Part model, mm, in its own coordinate system. Face numbers are marked on the shaded views. A direction names the side the tool comes from. Give positions to 0.01 mm unless a question says otherwise; leave off trailing zeros. Write each loop counter-clockwise with the first axis right and the second up, starting at its lowest first coordinate (ties: lowest second). Pieces come first, ordered by that corner, then holes. Notation, with made-up numbers: (57, 73.25) - (78, 73.25) arc R27 cw to (78, 91.25) - close; hole circle Ø3 at (55.5, 9.25). An arc over 180 degrees is marked (long way). Answer as a JSON object with one key per item and string values. Group by question number.
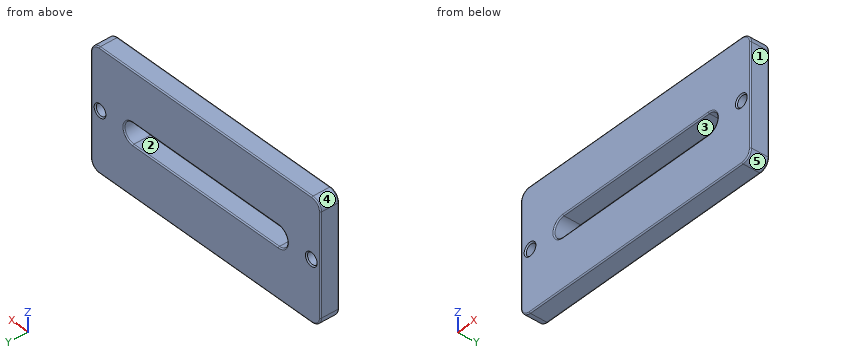
```python
from build123d import *

# Parameters (mm, degrees)
SKETCH1_W           = 82
SKETCH1_H           = 37.8
SKETCH1_R           = 1.75
BOSS_EXTRUDE1_DEPTH = 5.85
FILLET2_R           = 3
FILLET3_R           = 0.35
CHAMFER1_SIZE       = 0.35


with BuildPart() as part:
    # Sketch1 → Boss-Extrude1 (new body)
    with BuildSketch(Plane(origin=(0, 0, 0), x_dir=(1, 0, 0), z_dir=(0, 1, 0))):
        Rectangle(SKETCH1_W, SKETCH1_H)
        with Locations(Location((37.75, 0, 0), (0, 0, 270))):
            Circle(SKETCH1_R, mode=Mode.SUBTRACT)
        with Locations(Location((-37.75, 0, 0), (0, 0, 270))):
            Circle(SKETCH1_R, mode=Mode.SUBTRACT)
        with BuildLine():
            Line((-25.9975, 3.225), (-13.623486154, 3.225))
            Line((-13.623486154, 3.225), (13.623486154, 3.225))
            Line((13.623486154, 3.225), (25.9975, 3.225))
            ThreePointArc((25.9975, 3.225), (29.2225, 0), (25.9975, -3.225))
            Line((25.9975, -3.225), (13.623486154, -3.225))
            Line((13.623486154, -3.225), (-13.623486154, -3.225))
            Line((-13.623486154, -3.225), (-25.9975, -3.225))
            ThreePointArc((-25.9975, -3.225), (-29.2225, 0), (-25.9975, 3.225))
        make_face(mode=Mode.SUBTRACT)
    extrude(amount=BOSS_EXTRUDE1_DEPTH)

    # Fillet2
    fillet2_edges = [part.edges().sort_by_distance(p)[0] for p in [
        (-41, 2.925, -18.9),
        (41, 2.925, -18.9),
        (41, 2.925, 18.9),
        (-41, 2.925, 18.9),
    ]]
    fillet(fillet2_edges, radius=FILLET2_R)

    # Fillet3
    fillet3_edges = [part.edges().sort_by_distance(p)[0] for p in [
        (-29.2225, 0, 0),
        (0, 0, 3.225),
        (29.2225, 0, 0),
        (0, 0, -3.225),
        (0, 5.85, -3.225),
        (-29.2225, 5.85, 0),
        (0, 5.85, 3.225),
        (29.2225, 5.85, 0),
        (0, 0, -18.9),
        (0, 5.85, -18.9),
        (-41, 0, 0),
        (41, 0, 0),
        (0, 0, 18.9),
        (-40.121320344, 0, 18.021320344),
        (-40.121320344, 0, -18.021320344),
        (40.121320344, 0, 18.021320344),
        (40.121320344, 0, -18.021320344),
        (41, 5.85, 0),
        (-41, 5.85, 0),
        (0, 5.85, 18.9),
        (-40.121320344, 5.85, 18.021320344),
        (-40.121320344, 5.85, -18.021320344),
        (40.121320344, 5.85, 18.021320344),
        (40.121320344, 5.85, -18.021320344),
    ]]
    fillet(fillet3_edges, radius=FILLET3_R)

    # Chamfer1
    chamfer1_edges = [part.edges().sort_by_distance(p)[0] for p in [
        (37.75, 0, -1.75),
        (37.75, 5.85, -1.75),
        (-37.75, 0, -1.75),
        (-37.75, 5.85, -1.75),
    ]]
    chamfer(chamfer1_edges, length=CHAMFER1_SIZE)


solid = part.part
```
1) Band-saw the part on C-C (x = -2). List the corners of the cut face in (y, z) (3 decimals).
2) Mould opens along Z. For the marked faces 3, 4 and 5 say: pulls with the +Z half, pulls with the -Z half, needs draft (parallel to the pull), parting line crosses it, or undercut.
3) Band-saw the part on A-A (y = 4.6). State how many separate pieces and enclosed holes the cut face has, plus the area to 3 significant figures.
4) Drop flat-ended pins along their axis: P1, Ø3, axis at x = 37.75, z = 0, coming from the +Y side; P2, Ø4, axis at x = -37.75, z = 0, coming from the -Y side. Give the stop position or say it passes through.
5) Which spindle directions (+Z, -Z, +X, -X, +Y, -Y) get a long thin tool onto all of the face, cutting with end or side? Do the marked faces 1 and 2. Say none if no direction does.
6) Probe line 1 (X direction, y = 3.6, z = 0); line 2 (Z direction, x = -12, y = 4.25) (3 decimals); line 3 (X direction, y = 0.35, z = 1.5). List the from-to ranges inside material, lowest first.
Verdict:
{
 "1": {"outline": "(0, -18.55) arc R0.35 ccw to (0.35, -18.9) - (5.5, -18.9) arc R0.35 ccw to (5.85, -18.55) - (5.85, -3.575) arc R0.35 ccw to (5.5, -3.225) - (0.35, -3.225) arc R0.35 ccw to (0, -3.575) - close; (0, 3.575) arc R0.35 ccw to (0.35, 3.225) - (5.5, 3.225) arc R0.35 ccw to (5.85, 3.575) - (5.85, 18.55) arc R0.35 ccw to (5.5, 18.9) - (0.35, 18.9) arc R0.35 ccw to (0, 18.55) - close"},
 "2": {"face 3": "undercut", "face 4": "pulls with the +Z half", "face 5": "pulls with the -Z half"},
 "3": {"separate pieces": "1", "enclosed holes": "3", "area": "2,700 mm2"},
 "4": {"P1": "through", "P2": "y = 0.1"},
 "5": {"face 1": "+Z, -Z, +X, +Y, -Y", "face 2": "+Y, -Y"},
 "6": {"line 1": "-41 to -39.5, -36 to -29.22, 29.22 to 36, 39.5 to 41", "line 2": "-18.9 to -3.225, 3.225 to 18.9", "line 3": "-41 to -38.65, -36.85 to -28.85, 28.85 to 36.85, 38.65 to 41"}
}
